Autodesk Inventor part; units mm, degrees
ref_plane "YZ Plane" through (0, 0, 0) normal (1, 0, 0) x (0, 1, 0)
ref_plane "XZ Plane" through (0, 0, 0) normal (0, 1, 0) x (-1, 0, 0)
ref_plane "XY Plane" through (0, 0, 0) normal (0, 0, 1) x (1, 0, 0)
sketch "Sketch4" plane through (0, 0, 0) normal (0, 0, 1) x (1, 0, 0)
  circle A0 centre (0, 0) radius 2.5083
  circle A1 centre (0, 0) radius 3.9688
  line L0 (-3.9688, 0) -> (-3.9688, 12.7)
  arc A2 (-0.8259, 12.3821) -> (-3.9688, 12.7) centre (-2.3812, 12.7) ccw
  arc A3 (-0.8259, 12.3821) -> (2.5018, 3.0809) centre (8.5062, 10.475) ccw
  circle A4 centre (0, 0) radius 4.7625 construction
  circle A5 centre (15.7392, -2.0721) radius 6.35 construction
  circle A6 centre (15.7392, -2.0721) radius 3.9688
  circle A7 centre (15.7392, -2.0721) radius 1.7526
  line L1 (2.5018, 3.0809) -> (16.0883, 1.8813)
  circle A8 centre (6.35, -12.7) radius 3.9688
  circle A9 centre (6.35, -12.7) radius 1.7526
  line L2 (2.8002, -14.4749) -> (-3.5498, -1.7749)
  circle A10 centre (5.9564, -15.5682) radius 12.7
  line L3 (18.7135, -4.6997) -> (9.3243, -15.3276)
  line L4 (0, 0) -> (0, 4.7625) construction
  line L5 (0, 0) -> (15.7392, -2.0721) construction
  line L6 (15.7392, -2.0721) -> (16.2572, 1.8627) construction
  point P0 (3.9688, 0)
  point P1 (12.5559, -4.4423)
  point P2 (2.0561, -3.3946)
  point P3 (1.4182, -3.7067)
  point P4 (13.41, -5.2855)
  dimension "d54" = 9.525
  dimension "d44" = 5.0165
  dimension "d45" = 7.9375
  dimension "d51" = 12.7
  dimension "d52" = 3.175
  dimension "d53" = 9.525
  dimension "d56" = 12.7
  dimension "d57" = 7.9375
  dimension "d58" = 3.5052
  dimension "d61" = 7.9375
  dimension "d62" = 3.5052
  dimension "d63" = 12.7
  dimension "d64" = 6.35
  dimension "d67" = 97.5
  dimension "d68" = 15.875
  dimension "d69" = 25.4
extrude "Extrusion3" add sketch "Sketch4" along normal blind 7.9375 contours A1 | A1 L1 A6 A10 | A1 L0 A2 A3 | A6
fillet "Fillet5" radius 3.175 1 edges at (2.5018, 3.0809, 3.9688)
properties part number "Lever" material "Aluminum 6061"
Verification items for the finished model (mm, model axes). Coordinates: 2 decimals unless noted, no trailing zeros. Write each loop counter-clockwise with the first axis right and the second up, starting at its lowest first coordinate (ties: lowest second). Pieces come first, ordered by that corner, then holes. Notation, with made-up numbers: (57, 35) - (98, 35) arc R10 ccw to (98, 40) - close; hole circle Ø4 at (76, 50). An arc over 180 degrees is marked (long way). One line per question, with ' | ' between items. Start each with the question number.
1. Section check D-D (x = 0). Enter the section's corners in (y, z), plus the area to 3 significant figures.
2. Material ranges on line 1 along X through (y, z) = (-1, 4.75); line 2 along Y through (x, z) = (0, 4); line 3 along Y through (x, z) = (2.25, 3.25), recorded low to high.
3. Gauge pin test, flat ends, axial feed: P1, Ø3, axis at x = 0, y = 0, coming from the +Z side; P2, Ø1.5, axis at x = 2, z = 1, coming from the +Y side; P3, Ø2, axis at y = 2, z = 6, coming from the +X side; P4, Ø1, axis at y = 7, z = 5.5, coming from the +X side. Record the tip position at first contact, or that the pin passes through.
4. Section check A-A (y = -1). Enter the section's corners in (x, z).
5. Section check B-B (x = 15.25). Enter the section's corners in (y, z).
6. Section check C-C (z = 6). Count the separate pieces of the cut face and the enclosed holes in it, plus the area to 3 significant figures.
7. Draft check along X on faces 1 (the flat face through (-3.969, 6, 4)), 2 (the cylindrical face through (-2.205, -3.3, 3.913)), 3 (the flat face through (9.75, 2.44, 3.91)). Enter one of: released by +X, released by -X, zero draft, split by the parting line, or undercut.
Computed values:
1) outline: (-3.97, 0) - (-2.51, 0) - (-2.51, 7.94) - (-3.97, 7.94) - close; (2.51, 0) - (6.19, 0) - (6.19, 7.94) - (2.51, 7.94) - close | area: 40.8 mm²
2) line 1: -3.84 to -2.3, 2.3 to 14.35, 17.13 to 19.56 | line 2: -3.97 to -2.51, 2.51 to 6.19 | line 3: -3.42 to -1.11, 1.11 to 3.41
3) P1: through | P2: y = 4.3 | P3: x = 18.25 | P4: x = -0.15
4) outline: (-3.84, 0) - (-2.3, 0) - (-2.3, 7.94) - (-3.84, 7.94) - close; (2.3, 0) - (14.35, 0) - (14.35, 7.94) - (2.3, 7.94) - close; (17.13, 0) - (19.56, 0) - (19.56, 7.94) - (17.13, 7.94) - close
5) outline: (-6.01, 0) - (-3.76, 0) - (-3.76, 7.94) - (-6.01, 7.94) - close; (-0.39, 0) - (1.96, 0) - (1.96, 7.94) - (-0.39, 7.94) - close
6) separate pieces: 1 | enclosed holes: 2 | area: 162 mm²
7) face 1: released by -X | face 2: undercut | face 3: released by +X
